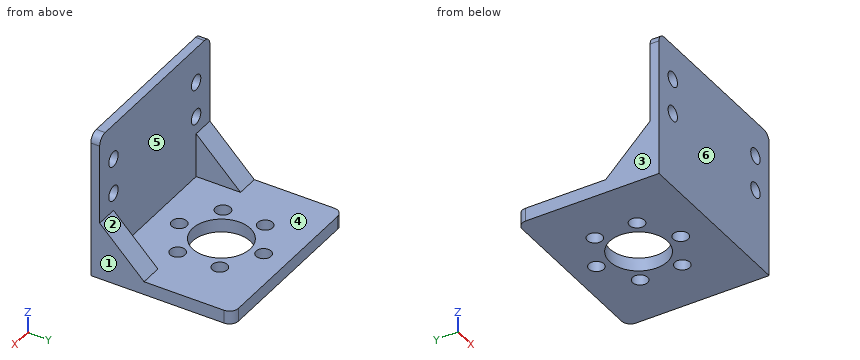
from build123d import *

# Parameters (mm, degrees)
SKETCH_2_W          = 40
SKETCH_2_H          = 32
SKETCH_2_R          = 1.7
EXTRUDE_2_DEPTH     = 3
CUT_EXTRUDE_1_REACH = 39.855
SKETCH_3_R          = 6.5
SKETCH_4_W          = 40
SKETCH_4_H          = 2
EXTRUDE_3_DEPTH     = 30
EXTRUDE_4_DEPTH     = 5
FILLET_1_R          = 2
SKETCH_6_R          = 1.7
CUT_EXTRUDE_2_DEPTH = 10


with BuildPart() as part:
    # 草图2 → 凸台-拉伸2 (new body)
    with BuildSketch(Plane.XY):
        with Locations((0, 16)):
            Rectangle(SKETCH_2_W, SKETCH_2_H)
        with Locations((0, 26.5)):
            Circle(SKETCH_2_R, mode=Mode.SUBTRACT)
        with Locations((8.227241336, 21.75)):
            Circle(SKETCH_2_R, mode=Mode.SUBTRACT)
        with Locations((8.227241336, 12.25)):
            Circle(SKETCH_2_R, mode=Mode.SUBTRACT)
        with Locations((0, 7.5)):
            Circle(SKETCH_2_R, mode=Mode.SUBTRACT)
        with Locations((-8.227241336, 12.25)):
            Circle(SKETCH_2_R, mode=Mode.SUBTRACT)
        with Locations((-8.227241336, 21.75)):
            Circle(SKETCH_2_R, mode=Mode.SUBTRACT)
    extrude(amount=EXTRUDE_2_DEPTH)

    # 草图3 → 切除-拉伸1 (cut, up to next)
    with BuildSketch(Plane.XY.offset(3), mode=Mode.PRIVATE) as cut_extrude_1_sk1:
        with Locations((0, 17)):
            Circle(SKETCH_3_R)
    cut_extrude_1_tool1 = extrude(cut_extrude_1_sk1.sketch, amount=-CUT_EXTRUDE_1_REACH, mode=Mode.PRIVATE) & part.part
    add(cut_extrude_1_tool1.solids().sort_by_distance((0, 17, 3))[0], mode=Mode.SUBTRACT)

    # 草图4 → 凸台-拉伸3 (add)
    with BuildSketch(Plane.XY.offset(3)):
        with Locations((0, 1)):
            Rectangle(SKETCH_4_W, SKETCH_4_H)
    extrude(amount=EXTRUDE_3_DEPTH)

    # 草图5 → 凸台-拉伸4 (add)
    with BuildSketch(Plane.ZY.offset(20)):
        Polygon((3, 12), (13, 2), (3, 2), align=None)
    extrude_4 = extrude(amount=-EXTRUDE_4_DEPTH)

    # 镜向1: 凸台-拉伸4 across plane
    add(extrude_4.mirror(Plane(origin=(0, 0, 0), x_dir=(0, 0, 1), z_dir=(1, 0, 0))))

    # 圆角1
    fillet_1_edges = [part.edges().sort_by_distance(p)[0] for p in [
        (-20, 1, 33),
        (20, 1, 33),
        (-20, 32, 1.5),
        (20, 32, 1.5),
    ]]
    fillet(fillet_1_edges, radius=FILLET_1_R)

    # 草图6 → 切除-拉伸2 (cut)
    with BuildSketch(Plane(origin=(0, 2, 0), x_dir=(1, 0, 0), z_dir=(0, 1, 0))):
        with Locations(Location((-15, -17, 0), (0, 0, 270))):
            Circle(SKETCH_6_R)
        with Locations(Location((15, -17, 0), (0, 0, 270))):
            Circle(SKETCH_6_R)
        with Locations(Location((-15, -25, 0), (0, 0, 270))):
            Circle(SKETCH_6_R)
        with Locations(Location((15, -25, 0), (0, 0, 270))):
            Circle(SKETCH_6_R)
    extrude(amount=-CUT_EXTRUDE_2_DEPTH, mode=Mode.SUBTRACT)


solid = part.part
Read the model definition and answer for the solid it produces. Units are mm, in the model's axes. Face numbers are marked on the shaded views. A direction names the side the tool comes from. Round coordinates to 2 decimals unless told otherwise and drop trailing zeros. Write each loop counter-clockwise with the first axis right and the second up, starting at its lowest first coordinate (ties: lowest second). Pieces come first, ordered by that corner, then holes.
1. The part is cut by section A-A, the plane y = 17. Determine the outline of the cut face in (x, z), then the cut area to 3 significant figures.
2. Straight lines are drawn through the part: L1, parallel to Y at x = 0, z = 1.5; L2, parallel to X at y = 1.4, z = 25; L3, parallel to Z at x = 13.5, y = 15. For each, find the intervals that lie inside material, in ascending order.
3. Given pin 1 Ø2 at (x, y) = (0, 26.5) entering from -Z; pin 2 Ø1 at (x, z) = (-3.5, 13.5) entering from +Y; pin 3 Ø4.5 at (x, y) = (-8.23, 21.75) entering from +Z, each flat-ended and moving along its own axis, determine where each tip first touches the part or whether it passes through.
4. The part is cut by section D-D, the plane z = 4. Determine the outline of the cut face in (x, y).
5. Which of the six approach directions +Z, -Z, +X, -X, +Y, -Y give full straight-line access (tool end or side, diameter ignored) to the marked faces 5 and 6?
6. The part is cut by section B-B, the plane z = 17. Determine the outline of the cut face in (x, y), then the cut area to 3 significant figures.
7. The part is cut by section C-C, the plane x = -14. Determine the outline of the cut face in (y, z).
8. Determine the mould class of the marked faces 1, 2, 3 and 4 for opening direction X: pulls with the +X half, pulls with the -X half, needs draft (parallel to the pull), parting line crosses it, or undercut.
Values:
1. outline: (-20, 0) - (-6.5, 0) - (-6.5, 3) - (-20, 3) - close; (6.5, 0) - (20, 0) - (20, 3) - (6.5, 3) - close
1. area: 81.0 mm2
2. L1: y = 0 to 5.8, 9.2 to 10.5, 23.5 to 24.8, 28.2 to 32
2. L2: x = -20 to -16.7, -13.3 to 13.3, 16.7 to 20
2. L3: z = 0 to 3
3. pin 1: passes through
3. pin 2: stops at y = 2
3. pin 3: stops at z = 3
4. outline: (-20, 0) - (20, 0) - (20, 11) - (15, 11) - (15, 2) - (-15, 2) - (-15, 11) - (-20, 11) - close
5. face 5: +Z, +Y
5. face 6: +Z, -Z, +X, -X, -Y
6. outline: (-20, 0) - (-16.7, 0) - (-16.7, 2) - (-20, 2) - close; (-13.3, 0) - (13.3, 0) - (13.3, 2) - (-13.3, 2) - close; (16.7, 0) - (20, 0) - (20, 2) - (16.7, 2) - close
6. area: 66.4 mm2
7. outline: (0, 0) - (32, 0) - (32, 3) - (2, 3) - (2, 15.63) - (0, 15.63) - close; (0, 18.37) - (2, 18.37) - (2, 23.63) - (0, 23.63) - close; (0, 26.37) - (2, 26.37) - (2, 33) - (0, 33) - close
8. face 1: pulls with the +X half
8. face 2: needs draft
8. face 3: pulls with the -X half
8. face 4: undercut
